Here's how the part is built. I have some questions about the finished solid (model axes, mm). Face numbers are marked on the shaded views. Give positions to 0.01 mm unless a question says otherwise; leave off trailing zeros. Write each loop counter-clockwise with the first axis right and the second up, starting at its lowest first coordinate (ties: lowest second). Pieces come first, ordered by that corner, then holes. Notation, with made-up numbers: (-21, 45.25) -> (33, 45.25) arc R31 cw to (33, 77.25) -> close; hole circle Ø1 at (-2, 88). An arc over 180 degrees is marked (long way). Use CSV: the item, a comma, the result in double quotes. Start each with the question number.
(1) Suppose I cut it at C-C on z = 0. List the corners of the cut face in (x, y) for me, plus the area to 3 significant figures.
(2) Suppose I cut it at A-A on x = 0. List the corners of the cut face in (y, z) for me.
(3) If we mould it in two halves opening along Z, with no side actions, what happens to the marked faces 1 and 2? For each: pulls with the +Z half, pulls with the -Z half, needs draft (parallel to the pull), parting line crosses it, or undercut.
(4) Suppose I cut it at D-D on z = -21.5. List the corners of the cut face in (x, y) for me, plus the area to 3 significant figures.
(5) For pin 1 Ø4 at (x, y) = (35, 14) entering from -Z; pin 2 Ø4 at (x, y) = (0, 10) entering from -Z; pin 3 Ø1 at (x, y) = (1, 8) entering from -Z; pin 4 Ø1 at (x, z) = (0, -43) entering from +Y, each with a flat end and sliding along its axis, tell me the tip position at first contact or that it passes through.
(6) I need wall thicknesses on L1, parallel to Y at x = -30.5, z = -30.5; L2, parallel to X at y = 20.5, z = 0; L3, parallel to Y at x = 0, z = -43.6. Which ranges of each line are inside material? Lowest first, please. Write a range as [from, to].
(7) Suppose I cut it at B-B on y = 10. Give the number of separate pieces and of enclosed holes in the cut face, plus the area to 3 significant figures.
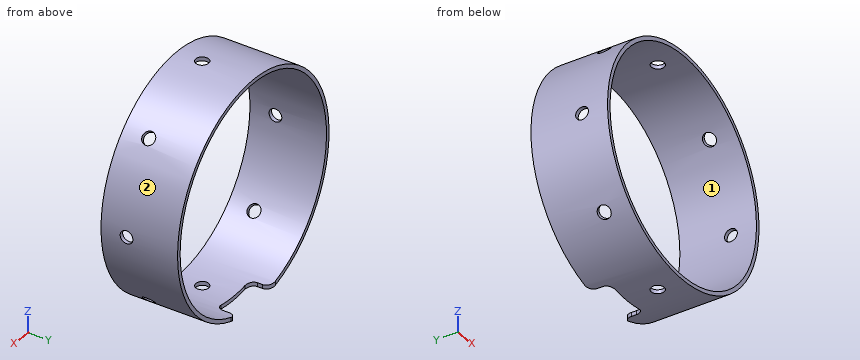
from build123d import *

# Parameters (mm, degrees)
SKIZZE1_R                       = 44.5
SKIZZE1_R_2                     = 43
AUFSATZ_LINEAR_AUSTRAGEN1_DEPTH = 30
SKIZZE3_R                       = 2.5
SCHNITT_LINEAR_AUSTRAGEN1_DEPTH = 45.5
KREISMUSTER1_COUNT              = 8
SCHNITT_LINEAR_AUSTRAGEN2_DEPTH = 45.500000122


with BuildPart() as part:
    # Skizze1 → Aufsatz-Linear austragen1 (new body)
    with BuildSketch(Plane(origin=(0, 0, 0), x_dir=(1, 0, 0), z_dir=(0, 1, 0))):
        Circle(SKIZZE1_R)
        Circle(SKIZZE1_R_2, mode=Mode.SUBTRACT)
    extrude(amount=AUFSATZ_LINEAR_AUSTRAGEN1_DEPTH)

    # Skizze3 → Schnitt-Linear austragen1 (cut, through all)
    with BuildSketch(Plane.XY):
        with Locations((0, 10)):
            Circle(SKIZZE3_R)
    schnitt_linear_austragen1 = extrude(amount=-SCHNITT_LINEAR_AUSTRAGEN1_DEPTH, mode=Mode.SUBTRACT)

    # Kreismuster1: Schnitt-Linear austragen1 ×8 about axis
    kreismuster1_axis = Axis((0, 30, 0), (0, -1, 0))
    for i in range(1, KREISMUSTER1_COUNT):
        add(schnitt_linear_austragen1.rotate(kreismuster1_axis, i * 360 / KREISMUSTER1_COUNT), mode=Mode.SUBTRACT)

    # Skizze4 → Schnitt-Linear austragen2 (cut, through all)
    with BuildSketch(Plane.XY):
        with BuildLine():
            Line((-13, 30), (13, 30))
            ThreePointArc((13, 30), (10.878679656, 29.121320344), (10, 27))
            Line((10, 27), (10, 25))
            ThreePointArc((10, 25), (9.121320344, 22.878679656), (7, 22))
            Line((7, 22), (-7, 22))
            ThreePointArc((-7, 22), (-9.121320344, 22.878679656), (-10, 25))
            Line((-10, 25), (-10, 27))
            ThreePointArc((-10, 27), (-10.878679656, 29.121320344), (-13, 30))
        make_face()
    extrude(amount=-SCHNITT_LINEAR_AUSTRAGEN2_DEPTH, mode=Mode.SUBTRACT)


solid = part.part
Geometry says:
1,outline,"(-44.5, 0) -> (-43, 0) -> (-43, 7.5) -> (-44.5, 7.5) -> close; (-44.5, 12.5) -> (-43, 12.5) -> (-43, 30) -> (-44.5, 30) -> close; (43, 0) -> (44.5, 0) -> (44.5, 7.5) -> (43, 7.5) -> close; (43, 12.5) -> (44.5, 12.5) -> (44.5, 30) -> (43, 30) -> close"
1,area,"75.0 mm²"
2,outline,"(0, -44.5) -> (7.5, -44.5) -> (7.5, -43) -> (0, -43) -> close; (0, 43) -> (7.5, 43) -> (7.5, 44.5) -> (0, 44.5) -> close; (12.5, -44.5) -> (22, -44.5) -> (22, -43) -> (12.5, -43) -> close; (12.5, 43) -> (30, 43) -> (30, 44.5) -> (12.5, 44.5) -> close"
3,face 1,"undercut"
3,face 2,"parting line crosses it"
4,outline,"(-38.96, 0) -> (-37.24, 0) -> (-37.24, 30) -> (-38.96, 30) -> close; (37.24, 0) -> (38.96, 0) -> (38.96, 30) -> (37.24, 30) -> close"
4,area,"103 mm²"
5,pin 1,"z = -29.85"
5,pin 2,"through"
5,pin 3,"z = -44.49"
5,pin 4,"y = 22"
6,L1,"[0, 7.5], [12.5, 30]"
6,L2,"[-44.5, -43], [43, 44.5]"
6,L3,"[0, 7.5], [12.5, 22]"
7,separate pieces,"8"
7,enclosed holes,"0"
7,area,"352 mm²"
